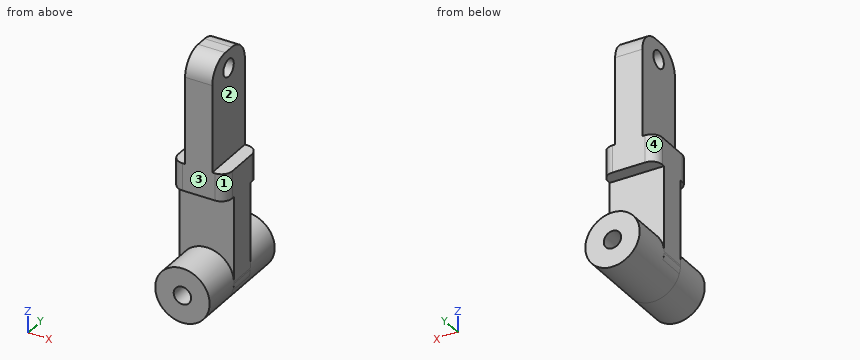
```python
from build123d import *

# Parameters (mm, degrees)
SKETCH_W          = 10
SKETCH_H          = 10
PAD_DEPTH         = 5
SKETCH001_W       = 5
SKETCH001_H       = 10
PAD001_DEPTH      = 20
SKETCH002_W       = 10
SKETCH002_H       = 5
PAD002_DEPTH      = 20
SKETCH003_R       = 1.6
POCKET_DEPTH      = 5
SKETCH004_R       = 1.6
POCKET001_DEPTH   = 7.501
FILLET_R          = 4
FILLET001_R       = 2
SKETCH006_R       = 5.00235
PAD003_DEPTH      = 7.5
PAD003_DEPTH_BACK = 12.5
SKETCH007_R       = 1.6
POCKET002_DEPTH   = 20.001


with BuildPart() as part:
    # Sketch → Pad (new body)
    with BuildSketch(Plane.XY):
        with Locations((-5, 5)):
            Rectangle(SKETCH_W, SKETCH_H)
    extrude(amount=PAD_DEPTH)

    # Sketch001 (on Face6 of Pad) → Pad001 (join)
    with BuildSketch(Plane.XY.offset(5)):
        with Locations((-5, 5)):
            Rectangle(SKETCH001_W, SKETCH001_H)
    extrude(amount=PAD001_DEPTH)

    # Sketch002 (on Face4 of Pad001) → Pad002 (join)
    with BuildSketch(Plane(origin=(0, 0, 0), x_dir=(1, 0, 0), z_dir=(0, 0, -1))):
        with Locations((-5, -5)):
            Rectangle(SKETCH002_W, SKETCH002_H)
    extrude(amount=PAD002_DEPTH)

    # Sketch003 (on Face17 of Pad002) → Pocket (cut)
    with BuildSketch(Plane(origin=(0, 7.5, 0), x_dir=(-1, 0, 0), z_dir=(0, 1, 0))):
        with Locations((5, -15.846688)):
            Circle(SKETCH003_R)
    extrude(amount=-POCKET_DEPTH, mode=Mode.SUBTRACT)

    # Sketch004 (on Face14 of Pocket) → Pocket001 (cut, through all)
    with BuildSketch(Plane(origin=(-7.5, 0, 0), x_dir=(0, -1, 0), z_dir=(-1, 0, 0))):
        with Locations((-5, 21.683375)):
            Circle(SKETCH004_R)
    extrude(amount=-POCKET001_DEPTH, mode=Mode.SUBTRACT)

    # Fillet
    fillet_edges = [part.edges().sort_by_distance(p)[0] for p in [
        (-10, 5, -20),
        (0, 5, -20),
        (-5, 10, 25),
        (-5, 0, 25),
    ]]
    fillet(fillet_edges, radius=FILLET_R)

    # Fillet001
    fillet001_edges = [part.edges().sort_by_distance(p)[0] for p in [
        (-10, 10, 2.5),
        (-10, 0, 2.5),
        (0, 10, 2.5),
        (0, 0, 2.5),
    ]]
    fillet(fillet001_edges, radius=FILLET001_R)

    # Sketch006 (on Face9 of Fillet001) → Pad003 (join, two sides)
    with BuildSketch(Plane.XZ.offset(-2.5)) as pad003_sk:
        with Locations((-5, -15.846688)):
            Circle(SKETCH006_R)
    extrude(amount=PAD003_DEPTH)
    extrude(pad003_sk.sketch, amount=-PAD003_DEPTH_BACK)

    # Sketch007 (on Face27 of Pad003) → Pocket002 (cut, through all)
    with BuildSketch(Plane.XZ.offset(5)):
        with Locations((-5, -15.846688)):
            Circle(SKETCH007_R)
    extrude(amount=-POCKET002_DEPTH, mode=Mode.SUBTRACT)


solid = part.part
```
Could you check a few things on this model? Use its own coordinates, in mm. Face numbers are marked on the shaded views. A direction names the side the tool comes from. Round coordinates to 2 decimals unless told otherwise and drop trailing zeros. Write each loop counter-clockwise with the first axis right and the second up, starting at its lowest first coordinate (ties: lowest second). Pieces come first, ordered by that corner, then holes.
(1) Suppose I cut it at B-B on y = 5. Write out the boundary of the cut face in (x, z).
Findings below:
outline: (-10, -16) arc R4 ccw to (-9.82, -17.2) arc R5 ccw to (-0.18, -17.2) arc R4 ccw to (0, -16) arc R5 ccw to (0, -15.69) - (0, 5) - (-2.5, 5) - (-2.5, 20.08) - (-7.5, 20.08) - (-7.5, 5) - (-10, 5) - (-10, -15.69) arc R5 ccw to start; (-7.5, 23.28) - (-2.5, 23.28) - (-2.5, 25) - (-7.5, 25) - close; hole circle Ø3.2 at (-5, -15.85)
(2) Suppose I cut it at A-A on x = -5. Write out the boundary of the cut face in (y, z), and give its area (3 significant figures).
Findings below:
outline: (-5, -20.85) - (15, -20.85) - (15, -17.45) - (-5, -17.45) - close; (-5, -14.25) - (15, -14.25) - (15, -10.84) - (7.5, -10.84) - (7.5, 0) - (10, 0) - (10, 21) arc R4 ccw to (6, 25) - (4, 25) arc R4 ccw to (0, 21) - (0, 0) - (2.5, 0) - (2.5, -10.84) - (-5, -10.84) - close; hole circle Ø3.2 at (5, 21.68)
area: 425 mm2
(3) For pin 1 (3 mm diameter, centred on y = 5.5, z = -3, fed in from +X); pin 2 (1.2 mm diameter, centred on x = -3, y = 8.5, fed in from -Z); pin 3 (3 mm diameter, centred on x = -3.5, z = 8.5, fed in from +Y); pin 4 (4 mm diameter, centred on x = -5, z = -15.85, fed in from -Y), each with a flat end and sliding along its axis, tell me the tip position at first contact or that it passes through.
Findings below:
pin 1: stops at x = 0
pin 2: stops at z = -20.65
pin 3: stops at y = 10
pin 4: stops at y = -5
(4) Suppose I cut it at C-C on z = 2.5. Write out the boundary of the cut face in (x, y), and give its area (3 significant figures).
Findings below:
outline: (-10, 2) arc R2 ccw to (-8, 0) - (-2, 0) arc R2 ccw to (0, 2) - (0, 8) arc R2 ccw to (-2, 10) - (-8, 10) arc R2 ccw to (-10, 8) - close
area: 96.6 mm2
(5) If I drill on probe 1 along Z at (x, y) = (-5, 5.25); probe 2 along Z at (x, y) = (-5, 0.5); probe 3 along Y at (x, z) = (-4, -2), over which ranges is the centre line in solid material (lowest first)?
Findings below:
probe 1: z = -20.85 to -17.45, -14.25 to 20.1, 23.26 to 25
probe 2: z = -20.85 to -17.45, -14.25 to -10.84, 0 to 22.94
probe 3: y = 2.5 to 7.5
(6) Which directions (+Z, -Z, +X, -X, +Y, -Y) give clear straight access to the entire face, cutting with the end or side of a thin tool? Please do the marked faces 1, 2, 3 and 4.
Findings below:
face 1: +Z, +X, -Y
face 2: +Z, +X, +Y, -Y
face 3: +Z, +X, -X, -Y
face 4: +Z, -X, +Y
(7) Suppose I cut it at D-D on y = -2.25. Write out the boundary of the cut face in (x, z).
Findings below:
outline: circle Ø10 at (-5, -15.85); hole circle Ø3.2 at (-5, -15.85)
